from build123d import *

# Parameters (mm, degrees)
EXTRUDE_1_DEPTH     = 1000
CUT_EXTRUDE_1_DEPTH = 46


with BuildPart() as part:
    # Эскиз1 → Вытянуть-Тонкостенный1 (new body)
    with BuildSketch(Plane(origin=(0, 0, 0), x_dir=(1, 0, 0), z_dir=(0, 1, 0))):
        Polygon((0, 45), (0, 0), (45, 0), (45, 5), (5, 5), (5, 45), align=None)
    extrude(amount=EXTRUDE_1_DEPTH)

    # Эскиз2 → Вырез-Вытянуть1 (cut, through all)
    with BuildSketch(Plane.ZY):
        Polygon((0, 0), (-45, 45), (-45, 0), align=None)
        Polygon((-45, 1000), (0, 1000), (-45, 955), align=None)
    extrude(amount=-CUT_EXTRUDE_1_DEPTH, mode=Mode.SUBTRACT)


solid = part.part
Input: part model. Units: mm. Frame: model coordinates. A direction names the side the tool comes from. Coordinates: 2 decimals unless noted, no trailing zeros. Loops run counter-clockwise (first coordinate to the right, second up) from the corner with the lowest first, then second, coordinate; pieces in that order, holes last. Notation, with made-up numbers: (40.25, -33) -> (50.25, -33) arc R12 cw to (50.25, -21) -> close; hole circle Ø7 at (-30, -13). An arc over 180 degrees is marked (long way). Write item = value, one per line. Start each with the question number.
Item 1: Cut plane A-A, the plane y = 495.5. Return loops of the section in (x, z).
Item 2: First-contact query: P1, Ø12, axis at x = 25, y = 439.5, coming from the -Z side; P2, Ø6, axis at y = 370, z = -21.5, coming from the +X side. Flat tips, straight axial feed; report the tip coordinate or a pass-through.
Item 3: Reachability of faces 1 (the face through (25, 493, -5)), 2 (the face through (4, 988, -12)) from +Z, -Z, +X, -X, +Y, -Y: full face, straight path, thin tool, end or side. Return the list, or none.
Item 4: Material intervals for line 1 (X direction, y = 535, z = -12); line 2 (Z direction, x = 13.5, y = 559); line 3 (Y direction, x = 4.5, z = -20), sorted ascending.
Item 5: Cut plane B-B, the plane z = -23. Return loops of the section in (x, y), plus the area to 3 significant figures.
Item 6: Cut plane C-C, the plane x = 12.5. Return loops of the section in (y, z).
Ans:
q1.outline = (0, -45) -> (5, -45) -> (5, -5) -> (45, -5) -> (45, 0) -> (0, 0) -> close
q2.P1 = -5
q2.P2 = 5
q3.face_1 = -Z, +X, +Y, -Y
q3.face_2 = -Z, +X, -X, +Y
q4.line_1 = 0 to 5
q4.line_2 = -5 to 0
q4.line_3 = 20 to 980
q5.outline = (0, 23) -> (5, 23) -> (5, 977) -> (0, 977) -> close
q5.area = 4,770 mm²
q6.outline = (0, 0) -> (5, -5) -> (995, -5) -> (1000, 0) -> close
